```python
from build123d import *

# Parameters (mm, degrees)
F2_R            = 3
F3_R            = 200
F5_D            = 10
F5_COPIES_COUNT = 10


# Not quite as in the source:
# - a pattern or mirror of a feature is missing from the dataset's text; its kind, count and spacing are read off the source's solid


with BuildPart() as f1:
    # F0 (on Front) → F1 (revolve)
    with BuildSketch(Plane.XZ):
        Polygon((-16.5, 133), (-16.5, 135), (-32.5, 135), (-32.5, 85), (-55.2756813566, 0), (-53.2051289958, 0), (-30.5, 84.7366950048), (-30.5, 133), align=None)
    revolve(axis=Axis((0, 0, 82.1189115205), (0, 0, -1)))

    # F2
    f2_edges = [f1.edges().sort_by_distance(p)[0] for p in [
        (32.5, 0, 135),
    ]]
    fillet(f2_edges, radius=F2_R)

    # F3
    f3_edges = [f1.edges().sort_by_distance(p)[0] for p in [
        (32.5, 0, 85),
    ]]
    fillet(f3_edges, radius=F3_R)

    # F5 (through all)
    with Locations(Plane.XY.offset(135)):
        with Locations((-10.2066846848, -21.7215005869)):
            f5 = Hole(F5_D / 2)

    # F5_copies: F5 ×10 about axis
    f5_copies_axis = Axis((0, 0, 0), (0, 0, 1))
    for i in range(1, F5_COPIES_COUNT):
        add(f5.rotate(f5_copies_axis, i * 360 / F5_COPIES_COUNT), mode=Mode.SUBTRACT)


solid = f1.part
```
Check sheet for the modelled part. Datum: model origin and axes. Units: mm. A direction names the side the tool comes from. Give positions to 0.01 mm unless a question says otherwise; leave off trailing zeros. Write each loop counter-clockwise with the first axis right and the second up, starting at its lowest first coordinate (ties: lowest second). Pieces come first, ordered by that corner, then holes.
Item 1: Cross-section at D-D (z = 30). Enter the section's corners in (x, y).
Item 2: Cross-section at B-B (y = 0). Count the separate pieces of the cut face and the enclosed holes in it, and give its area (3 significant figures).
Item 3: Access from +Z, -Z, +X, -X, +Y, -Y to the whole of each face (thin tool, end or side, straight path). Record for faces 1 (the face through (29, 45, 0)), 2 (the face through (16, 5, 133)), 3 (the face through (-31, 9.76, 121.52)).
Item 4: Cross-section at A-A (z = 122). Enter the section's corners in (x, y), and give its area (3 significant figures).
Item 5: Draft check along Z on faces 4 (the face through (8.49, -38.24, 52.38)), 5 (the face through (-21.624, 13.586, 133.986)), 6 (the face through (-41.835, 13.174, 42.603)). Enter one of: released by +Z, released by -Z, zero draft, split by the parting line, or undercut.
Item 6: Gauge pin test, flat ends, axial feed: pin 1 (5 mm diameter, centred on y = 42, z = 19, fed in from +X); pin 2 (4 mm diameter, centred on y = 10.5, z = 72, fed in from -X); pin 3 (5 mm diameter, centred on y = -5, z = 115, fed in from +X); pin 4 (6 mm diameter, centred on x = -10.21, y = -21.72, fed in from -Z). Record the tip position at first contact, or that the pin passes through.
Item 7: Scan lines: L1, parallel to Y at x = -2.5, z = 6.5; L2, parallel to Y at x = -17, z = 75; L3, parallel to X at y = -6, z = 129. Record each from-to range of solid material in increasing order.
Report:
1. outline: circle Ø94.47 at (0, 0); hole circle Ø90.33 at (0, 0)
2. separate pieces: 4
2. enclosed holes: 0
2. area: 632 mm2
3. face 1: -Z, +X, -X, +Y, -Y
3. face 2: -Z
3. face 3: +Z
4. outline: circle Ø65 at (0, 0); hole circle Ø61 at (0, 0)
4. area: 396 mm2
5. face 4: released by -Z
5. face 5: zero draft
5. face 6: released by +Z
6. pin 1: stops at x = 31.14
6. pin 2: stops at x = -35.55
6. pin 3: stops at x = 32.4
6. pin 4: passes through
7. L1: y = -53.48 to -51.4, 51.4 to 53.48
7. L2: y = -31.54 to -28.41, 28.41 to 31.54
7. L3: x = -31.94 to -29.9, 29.9 to 31.94
